from build123d import *

# Parameters (mm, degrees)
SKETCH1_R           = 20.32
BOSS_EXTRUDE1_DEPTH = 21.59
SKETCH2_W           = 15.24
SKETCH2_H           = 4.318
SKETCH3_W           = 5.08
SKETCH3_H           = 14.732
CUT_EXTRUDE1_REACH  = 37.943
SKETCH4_R           = 1.27
CIRPATTERN1_COUNT   = 6
CUT_EXTRUDE2_REACH  = 37.943
SKETCH5_R           = 4.699
SKETCH9_R           = 1.905
CUT_EXTRUDE3_DEPTH  = 51.305467894


with BuildPart() as part:
    # Sketch1 → Boss-Extrude1 (new body)
    with BuildSketch(Plane(origin=(0, 0, 0), x_dir=(1, 0, 0), z_dir=(0, 1, 0))):
        with Locations(Location((0, 0, 0), (0, 0, 270))):
            Circle(SKETCH1_R)
    extrude(amount=BOSS_EXTRUDE1_DEPTH)

    # Sketch2 → Cut-Revolve1 (revolve, cut)
    with BuildSketch(Plane.XY, mode=Mode.PRIVATE) as cut_revolve1_sk:
        with Locations((-7.62, 19.431)):
            Rectangle(SKETCH2_W, SKETCH2_H)
    revolve(cut_revolve1_sk.sketch.rotate(Axis((0, 55, 0), (0, -1, 0)), 270), axis=Axis((0, 55, 0), (0, -1, 0)), mode=Mode.SUBTRACT)

    # Sketch3 → Cut-Revolve2 (revolve, cut)
    with BuildSketch(Plane.XY, mode=Mode.PRIVATE) as cut_revolve2_sk:
        with Locations((-17.78, 7.366)):
            Rectangle(SKETCH3_W, SKETCH3_H)
    revolve(cut_revolve2_sk.sketch.rotate(Axis((0, 55, 0), (0, -1, 0)), 270), axis=Axis((0, 55, 0), (0, -1, 0)), mode=Mode.SUBTRACT)

    # Sketch4 → Cut-Extrude1 (cut, up to next)
    with BuildSketch(Plane(origin=(0, 21.59, 0), x_dir=(1, 0, 0), z_dir=(0, 1, 0)), mode=Mode.PRIVATE) as cut_extrude1_sk1:
        with Locations(Location((0, 17.78, 0), (0, 0, 270))):
            Circle(SKETCH4_R)
    cut_extrude1_tool1 = extrude(cut_extrude1_sk1.sketch, amount=-CUT_EXTRUDE1_REACH, mode=Mode.PRIVATE) & part.part
    cut_extrude1 = cut_extrude1_tool1.solids().sort_by_distance((0, 21.59, -17.78))[0]
    add(cut_extrude1, mode=Mode.SUBTRACT)

    # CirPattern1: Cut-Extrude1 ×6 about axis
    cirpattern1_axis = Axis((0, 0, 0), (0, 1, 0))
    for i in range(1, CIRPATTERN1_COUNT):
        add(cut_extrude1.rotate(cirpattern1_axis, i * 360 / CIRPATTERN1_COUNT), mode=Mode.SUBTRACT)

    # Sketch5 → Cut-Extrude2 (cut, up to next)
    with BuildSketch(Plane.XZ, mode=Mode.PRIVATE) as cut_extrude2_sk1:
        with Locations(Location((0, 0, 0), (0, 0, 270))):
            Circle(SKETCH5_R)
    cut_extrude2_tool1 = extrude(cut_extrude2_sk1.sketch, amount=-CUT_EXTRUDE2_REACH, mode=Mode.PRIVATE) & part.part
    add(cut_extrude2_tool1.solids().sort_by_distance((0, 0, 0))[0], mode=Mode.SUBTRACT)

    # Sketch7 → Cut-Revolve3 (revolve, cut)
    with BuildSketch(Plane.XY, mode=Mode.PRIVATE) as cut_revolve3_sk:
        Polygon((-15.24, 14.732), (-11.40968, 10.90168), (-11.40968, 0), (-15.24, 0), align=None)
    revolve(cut_revolve3_sk.sketch.rotate(Axis((0, 55, 0), (0, -1, 0)), 270), axis=Axis((0, 55, 0), (0, -1, 0)), mode=Mode.SUBTRACT)

    # Sketch8 → Cut-Revolve4 (revolve, cut)
    with BuildSketch(Plane.XY, mode=Mode.PRIVATE) as cut_revolve4_sk:
        Polygon((-4.699, 17.272), (-13.97, 17.272), (-13.97, 16.002), (-4.699, 6.731), align=None)
    revolve(cut_revolve4_sk.sketch.rotate(Axis((0, 55, 0), (0, -1, 0)), 270), axis=Axis((0, 55, 0), (0, -1, 0)), mode=Mode.SUBTRACT)

    # Sketch9 → Cut-Extrude3 (cut, through all)
    with BuildSketch(Plane(origin=(20.32, 0, 0), x_dir=(0, 0, -1), z_dir=(1, 0, 0))):
        with Locations((0, 21.59)):
            Circle(SKETCH9_R)
    extrude(amount=-CUT_EXTRUDE3_DEPTH, mode=Mode.SUBTRACT)


solid = part.part
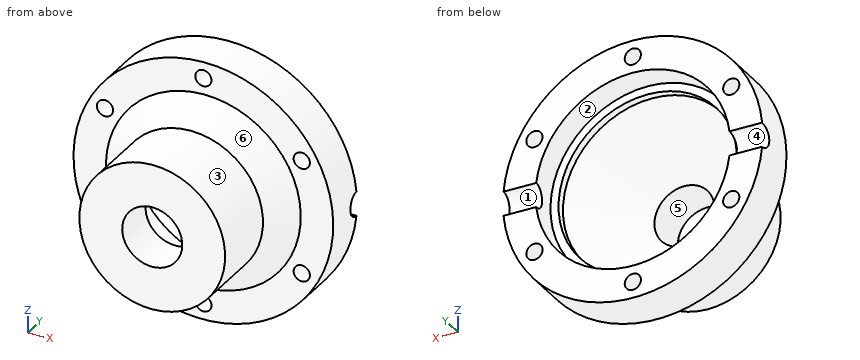
The listing builds one solid part. Answer for the finished solid, in the listing's coordinates (mm). Face numbers are marked on the shaded views. A direction names the side the tool comes from. Coordinates: 2 decimals unless noted, no trailing zeros. Order: outer loops, then holes, each group sorted by start corner. A loop starts at its lowest first (then second) coordinate and runs counter-clockwise, first axis right, second up.
Q1. A cutting plane is placed at B-B, the plane x = 0. State how many separate pieces and enclosed holes the cut face has, and give its area (3 significant figures).
Q2. Given P1, Ø1.5, axis at x = -12, z = 11.5, coming from the -Y side; P2, Ø1.5, axis at x = 3, y = 4, coming from the +Z side; P3, Ø5, axis at y = 4, z = 4, coming from the -X side; P4, Ø20.5, axis at x = 6, z = -5.5, coming from the -Y side, each flat-ended and moving along its own axis, determine where each tip first touches the part or whether it passes through.
Q3. A cutting plane is placed at A-A, the plane z = 0. Write down the section's boundary in (x, y) (3 decimals).
Q4. A cutting plane is placed at C-C, the plane x = -16. Write down the section's boundary in (y, z) (3 decimals), and give its area (3 significant figures).
Q5. For a pull along X with two mould halves and no side action, classify the marked faces 4, 5 and 6 as pulls with the +X half, pulls with the -X half, needs draft (parallel to the pull), parting line crosses it, or undercut.
Q6. A cutting plane is placed at D-D, the plane z = -17.78. Write down the section's boundary in (x, y).
Q7. Consider line 1 (X direction, y = 18.75, z = -8.89); line 2 (Y direction, x = 15, z = -12); line 3 (X direction, y = 1.75, z = 0). Determine where each line is inside the solid, lowest interval first.
Q8. Which of the six approach directions +Z, -Z, +X, -X, +Y, -Y give full straight-line access (tool end or side, diameter ignored) to the marked faces 1, 2 and 3?
Answers follow:
1. separate pieces: 4
1. enclosed holes: 0
1. area: 191 mm2
2. P1: stops at y = 14.73
2. P2: stops at z = 11.19
2. P3: stops at x = -11.31
2. P4: stops at y = 0
3. outline: (-20.32, 14.732) - (-15.24, 14.732) - (-11.41, 10.902) - (-11.41, 0) - (-4.699, 0) - (-4.699, 6.731) - (-13.97, 16.002) - (-13.97, 17.272) - (-15.24, 17.272) - (-15.24, 19.685) - (-20.32, 19.685) - close; (4.699, 0) - (11.41, 0) - (11.41, 10.902) - (15.24, 14.732) - (20.32, 14.732) - (20.32, 19.685) - (15.24, 19.685) - (15.24, 17.272) - (13.97, 17.272) - (13.97, 16.002) - (4.699, 6.731) - close
4. outline: (14.732, -12.526) - (21.59, -12.526) - (21.59, -10.008) - (14.732, -10.008) - close; (14.732, -7.772) - (21.59, -7.772) - (21.59, -1.905) arc R1.905 cw to (21.59, 1.905) - (21.59, 7.772) - (14.732, 7.772) - close; (14.732, 10.008) - (21.59, 10.008) - (21.59, 12.526) - (14.732, 12.526) - close
4. area: 135 mm2
5. face 4: needs draft
5. face 5: undercut
5. face 6: parting line crosses it
6. outline: (-9.84, 14.73) - (-1.27, 14.73) - (-1.27, 21.59) - (-9.84, 21.59) - close; (1.27, 14.73) - (9.84, 14.73) - (9.84, 21.59) - (1.27, 21.59) - close
7. line 1: x = -18.27 to -16.67, -14.13 to -12.38, 12.38 to 14.13, 16.67 to 18.27
7. line 2: y = 14.73 to 21.59
7. line 3: x = -11.41 to -4.7, 4.7 to 11.41
8. face 1: +X, -X, +Y
8. face 2: +Y
8. face 3: -Y
